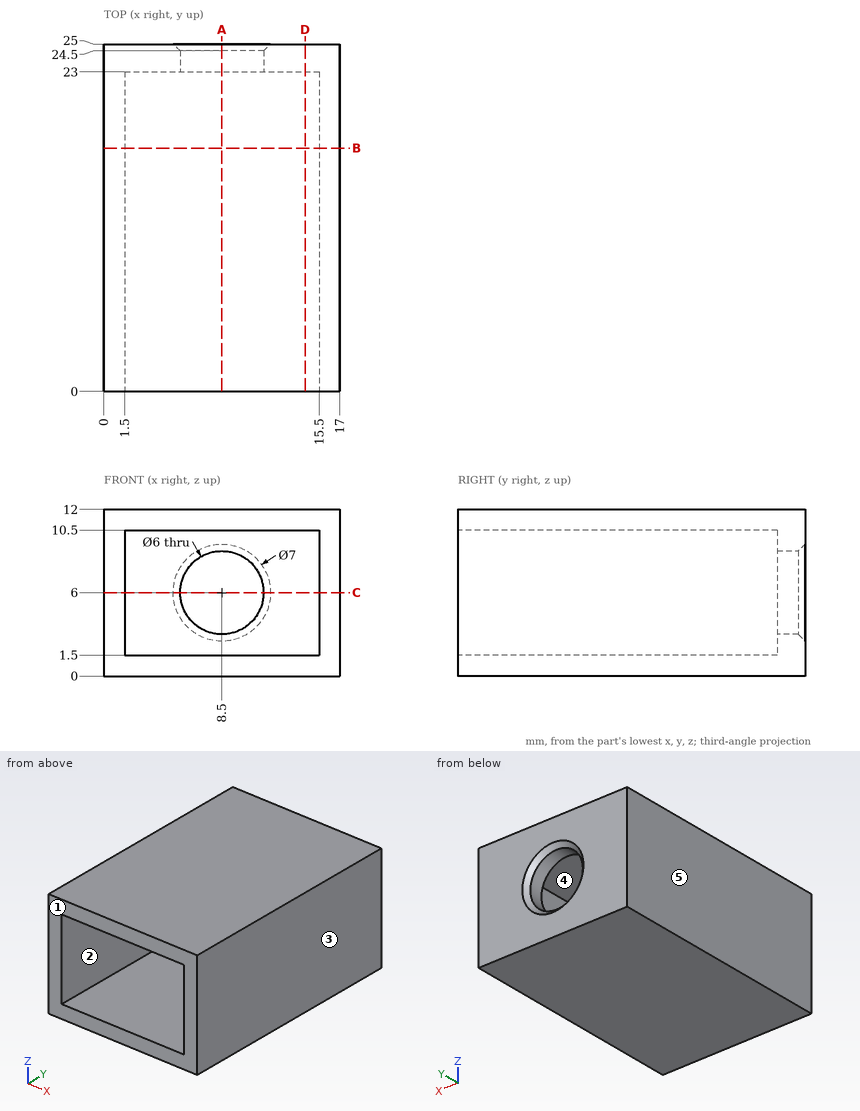
Study the drawing (mm; zero at the part's minimum x, y, z) and answer. A direction names the side the tool comes from. Give positions to 0.01 mm unless a question says otherwise; leave off trailing zeros. Order: outer loops, then holes, each group sorted by start corner. A loop starts at its lowest first (then second) coordinate and runs counter-clockwise, first axis right, second up.
1) Determine the mould class of the marked faces 1, 2 and 3 for opening direction X: pulls with the +X half, pulls with the -X half, needs draft (parallel to the pull), parting line crosses it, or undercut.
Reported:
face 1: needs draft
face 2: undercut
face 3: pulls with the +X half
2) Given P1, Ø2, axis at x = 7, z = 8, coming from the -Y side; P2, Ø5.5, axis at x = 8.5, z = 6, coming from the -Y side, each flat-ended and moving along its own axis, determine where each tip first touches the part or whether it passes through.
Reported:
P1: stops at y = 23
P2: passes through
3) Consider line 1 along Z through (x, y) = (4.5, 21.75); line 2 along X through (y, z) = (23.65, 6); line 3 along X through (y, z) = (16.5, 7.5). Determine where each line is inside the solid, lowest interval first.
Reported:
line 1: z = 0 to 1.5, 10.5 to 12
line 2: x = 0 to 5.5, 11.5 to 17
line 3: x = 0 to 1.5, 15.5 to 17
4) Find section D-D on x = 14.5. Write down the section's boundary in (y, z).
Reported:
outline: (0, 0) - (25, 0) - (25, 12) - (0, 12) - (0, 10.5) - (23, 10.5) - (23, 1.5) - (0, 1.5) - close
5) Find section B-B on y = 17.5. Write down the section's boundary in (x, z).
Reported:
outline: (0, 0) - (17, 0) - (17, 12) - (0, 12) - close; hole (1.5, 1.5) - (15.5, 1.5) - (15.5, 10.5) - (1.5, 10.5) - close
6) Find section A-A on x = 8.5. Write down the section's boundary in (y, z), then the cut area to 4 significant figures.
Reported:
outline: (0, 0) - (25, 0) - (25, 2.5) - (24.5, 3) - (23, 3) - (23, 1.5) - (0, 1.5) - close; (0, 10.5) - (23, 10.5) - (23, 9) - (24.5, 9) - (25, 9.5) - (25, 12) - (0, 12) - close
area: 80.75 mm2
7) Find section C-C on z = 6. Write down the section's boundary in (x, y).
Reported:
outline: (0, 0) - (1.5, 0) - (1.5, 23) - (5.5, 23) - (5.5, 24.5) - (5, 25) - (0, 25) - close; (11.5, 23) - (15.5, 23) - (15.5, 0) - (17, 0) - (17, 25) - (12, 25) - (11.5, 24.5) - close
8) For the marked faces 4 and 5, determine the directions among +Z, -Z, +X, -X, +Y, -Y from which every point of the face is accessible in a straight line to the end or side of a thin tool.
Reported:
face 4: -Y
face 5: +Z, -Z, -X, +Y, -Y
